Verification items for the finished model (mm, model axes). A direction names the side the tool comes from. Give positions to 0.01 mm unless a question says otherwise; leave off trailing zeros. Write each loop counter-clockwise with the first axis right and the second up, starting at its lowest first coordinate (ties: lowest second). Pieces come first, ordered by that corner, then holes.
from build123d import *

# Parameters (mm, degrees)
F1_DEPTH      = 8.5
F1_DEPTH_BACK = 12.5
F2_R          = 2.6
F3_DEPTH      = 13
F3_DEPTH_BACK = 13
F4_R          = 2.6
F5_DEPTH      = 25
F5_DEPTH_BACK = 25
F6_SIZE       = 12
F7_R          = 1


with BuildPart() as f1:
    # F0 (on Front) → F1 (new body, two sides)
    with BuildSketch(Plane.XZ) as f1_sk:
        Polygon((4.5, 15.5), (-3.5, 15.5), (-3.5, 3.5), (-13.7, 3.5), (-13.7, 15.5), (-21.7, 15.5), (-21.7, -4.5), (4.5, -4.5), align=None)
    extrude(amount=F1_DEPTH)
    extrude(f1_sk.sketch, amount=-F1_DEPTH_BACK)

    # F2 (on Front) → F3 (cut, two sides)
    with BuildSketch(Plane.XZ) as f3_sk:
        Circle(F2_R)
        with Locations((-17.2, 0)):
            Circle(F2_R)
    extrude(amount=F3_DEPTH, mode=Mode.SUBTRACT)
    extrude(f3_sk.sketch, amount=-F3_DEPTH_BACK, mode=Mode.SUBTRACT)

    # F4 (on Right) → F5 (cut, two sides)
    with BuildSketch(Plane.YZ) as f5_sk:
        with Locations((8, 11)):
            Circle(F4_R)
    extrude(amount=-F5_DEPTH, mode=Mode.SUBTRACT)
    extrude(f5_sk.sketch, amount=F5_DEPTH_BACK, mode=Mode.SUBTRACT)

    # F6
    f6_edges = [f1.edges().sort_by_distance(p)[0] for p in [
        (-17.7, -8.5, 15.5),
        (0.5, -8.5, 15.5),
    ]]
    chamfer(f6_edges, length=F6_SIZE)

    # F7
    f7_edges = [f1.edges().sort_by_distance(p)[0] for p in [
        (4.5, 2, -4.5),
        (4.5, 8, 15.5),
        (-21.7, 2, -4.5),
        (-21.7, 8, 15.5),
        (-13.7, 8, 15.5),
        (-3.5, 2, 3.5),
        (-13.7, 2, 3.5),
        (-3.5, 8, 15.5),
    ]]
    fillet(f7_edges, radius=F7_R)


solid = f1.part
Item 1: Sectioned sample at C-C on z = 11. Record the cut outline in (x, y).
Answer key:
outline: (-21.7, -1) - (-13.7, -1) - (-13.7, 5.4) - (-21.7, 5.4) - close; (-21.7, 10.6) - (-13.7, 10.6) - (-13.7, 12.5) - (-21.7, 12.5) - close; (-3.5, -1) - (4.5, -1) - (4.5, 5.4) - (-3.5, 5.4) - close; (-3.5, 10.6) - (4.5, 10.6) - (4.5, 12.5) - (-3.5, 12.5) - close
Item 2: Sectioned sample at A-A on x = 0. Record the cut outline in (y, z).
Answer key:
outline: (-8.5, -4.5) - (12.5, -4.5) - (12.5, -2.6) - (-8.5, -2.6) - close; (-8.5, 2.6) - (12.5, 2.6) - (12.5, 15.5) - (3.5, 15.5) - (-8.5, 3.5) - close; hole circle Ø5.2 at (8, 11)
Item 3: Sectioned sample at D-D on z = 0. Record the cut outline in (x, y).
Answer key:
outline: (-21.7, -8.5) - (-19.8, -8.5) - (-19.8, 12.5) - (-21.7, 12.5) - close; (-14.6, -8.5) - (-2.6, -8.5) - (-2.6, 12.5) - (-14.6, 12.5) - close; (2.6, -8.5) - (4.5, -8.5) - (4.5, 12.5) - (2.6, 12.5) - close
Item 4: Set-up check for faces 1 (the face through (-21.415, 7.43, 15.199)), 2 (the face through (-13.399, 1.853, 3.785)): record each of +Z, -Z, +X, -X, +Y, -Y from which the full face is reachable in a straight line by a thin tool's end or side.
Answer key:
face 1: +Z, -X, +Y, -Y
face 2: +Z, +Y, -Y
Item 5: Sectioned sample at B-B on y = -4.25. Record the cut outline in (x, z), then the cut area to 3 significant figures.
Answer key:
outline: (-21.7, -3.5) arc R1 ccw to (-20.7, -4.5) - (3.5, -4.5) arc R1 ccw to (4.5, -3.5) - (4.5, 7.75) - (-3.5, 7.75) - (-3.5, 4.5) arc R1 cw to (-4.5, 3.5) - (-12.7, 3.5) arc R1 cw to (-13.7, 4.5) - (-13.7, 7.75) - (-21.7, 7.75) - close; hole circle Ø5.2 at (-17.2, 0); hole circle Ø5.2 at (0, 0)
area: 235 mm2
Item 6: Release check for a two-part mould opening along Z. For faces 3 (the face through (-18, 8, 15.5)), 4 (the face through (-17.644, 9.2, 8.693)), 5 (the face through (-21.399, 2.147, -4.215)) record: released by +Z, released by -Z, zero draft, split by the parting line, or undercut.
Answer key:
face 3: released by +Z
face 4: undercut
face 5: released by -Z
Item 7: Scan lines: line 1 along X through (y, z) = (7.25, 0); line 2 along Z through (x, y) = (-17.2, 8); line 3 along Z through (x, y) = (-0.5, 9). Record each from-to range of solid material in increasing order.
Answer key:
line 1: x = -21.7 to -19.8, -14.6 to -2.6, 2.6 to 4.5
line 2: z = -4.5 to -2.6, 2.6 to 8.4, 13.6 to 15.5
line 3: z = -4.5 to -2.55, 2.55 to 8.6, 13.4 to 15.5
Item 8: Depth check by flat-ended pin: pin 1 (4 mm diameter, centred on x = -9, y = 4, fed in from +Z); pin 2 (4.5 mm diameter, centred on x = -17.2, z = 0, fed in from -Y). Enter the tip coordinate at first touch or a pass-through.
Answer key:
pin 1: stops at z = 3.5
pin 2: passes through
